Answer from the drawing. Dimensions are ordinates in mm from the lowest x, y and z of the part. A direction names the side the tool comes from. Round coordinates to 2 decimals unless told otherwise and drop trailing zeros. Write each loop counter-clockwise with the first axis right and the second up, starting at its lowest first coordinate (ties: lowest second). Pieces come first, ordered by that corner, then holes. Notation, with made-up numbers: (25, 38) - (84, 38) arc R14 ccw to (84, 46) - close; hole circle Ø5 at (-20.75, 59). An arc over 180 degrees is marked (long way). Answer in a Markdown table with one row per item.
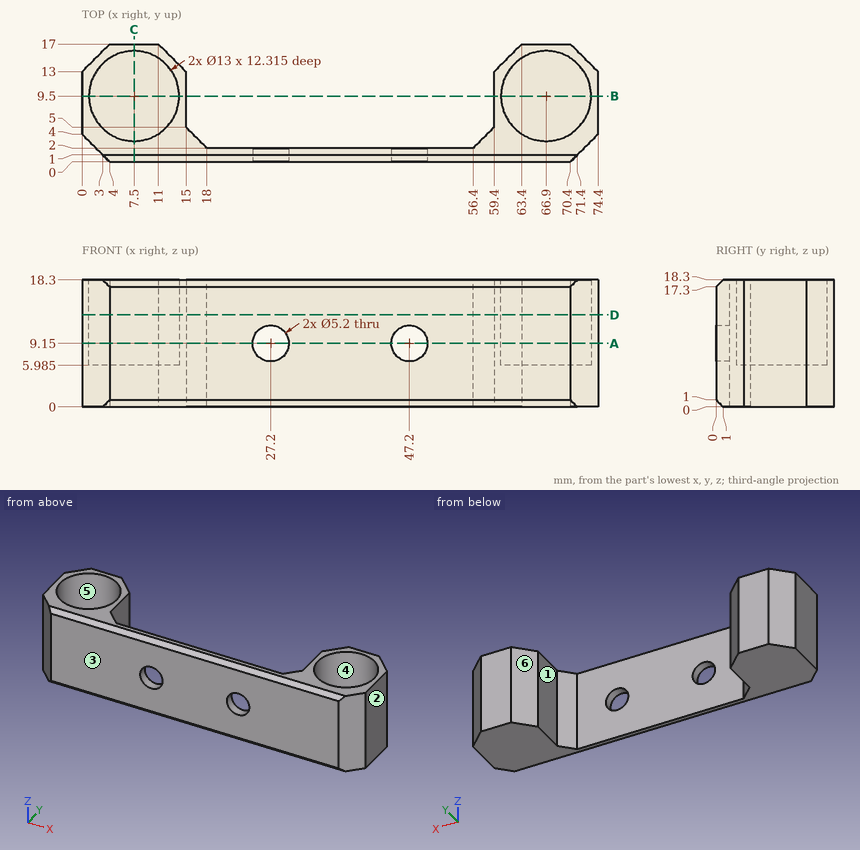
(1) For the marked faces 1 and 2, determine the directions among +Z, -Z, +X, -X, +Y, -Y from which every point of the face is accessible in a straight line to the end or side of a thin tool.
Checked values:
| item | result |
|---|---|
| face 1 | +Z, -Z, +Y |
| face 2 | +Z, -Z, +X, +Y, -Y |
(2) Section D-D (z = 13.25) is taken. Give the vertices of the cut face in (x, y), and give its area (3 significant figures).
Checked values:
| item | result |
|---|---|
| outline | (0, 4) - (4, 0) - (70.4, 0) - (74.4, 4) - (74.4, 13) - (70.4, 17) - (63.4, 17) - (59.4, 13) - (59.4, 5) - (56.4, 2) - (18, 2) - (15, 5) - (15, 13) - (11, 17) - (4, 17) - (0, 13) - close; hole circle Ø13 at (7.5, 9.5); hole circle Ø13 at (66.9, 9.5) |
| area | 294 mm2 |
(3) For a pull along Y with two mould halves and no side action, classify the marked faces 3, 4, 5 and 6 as pulls with the +Y half, pulls with the -Y half, needs draft (parallel to the pull), parting line crosses it, or undercut.
Checked values:
| item | result |
|---|---|
| face 3 | pulls with the -Y half |
| face 4 | undercut |
| face 5 | undercut |
| face 6 | pulls with the +Y half |
(4) Section B-B (y = 9.5) is taken. Give the vertices of the cut face in (x, z) (3 decimals), and give its area (3 significant figures).
Checked values:
| item | result |
|---|---|
| outline | (0, 0) - (15, 0) - (15, 18.3) - (14, 18.3) - (14, 5.985) - (1, 5.985) - (1, 18.3) - (0, 18.3) - close; (59.4, 0) - (74.4, 0) - (74.4, 18.3) - (73.4, 18.3) - (73.4, 5.985) - (60.4, 5.985) - (60.4, 18.3) - (59.4, 18.3) - close |
| area | 229 mm2 |
(5) Section A-A (z = 9.15) is taken. Give the vertices of the cut face in (x, y), and give its area (3 significant figures).
Checked values:
| item | result |
|---|---|
| outline | (0, 4) - (4, 0) - (24.6, 0) - (24.6, 2) - (18, 2) - (15, 5) - (15, 13) - (11, 17) - (4, 17) - (0, 13) - close; (29.8, 0) - (44.6, 0) - (44.6, 2) - (29.8, 2) - close; (49.8, 0) - (70.4, 0) - (74.4, 4) - (74.4, 13) - (70.4, 17) - (63.4, 17) - (59.4, 13) - (59.4, 5) - (56.4, 2) - (49.8, 2) - close; hole circle Ø13 at (7.5, 9.5); hole circle Ø13 at (66.9, 9.5) |
| area | 274 mm2 |
(6) Find the intervals of material crossed by line 1 (X direction, y = 5.5, z = 12); line 2 (X direction, y = 6.25, z = 12.25); line 3 (X direction, y = 0.95, z = 9.15), in increasing order.
Checked values:
| item | result |
|---|---|
| line 1 | x = 0 to 2.38, 12.62 to 15, 59.4 to 61.78, 72.02 to 74.4 |
| line 2 | x = 0 to 1.87, 13.13 to 15, 59.4 to 61.27, 72.53 to 74.4 |
| line 3 | x = 3.05 to 24.6, 29.8 to 44.6, 49.8 to 71.35 |
(7) Section C-C (x = 7.5) is taken. Give the vertices of the cut face in (y, z) (3 decimals), and give its area (3 significant figures).
Checked values:
| item | result |
|---|---|
| outline | (0, 1) - (1, 0) - (17, 0) - (17, 18.3) - (16, 18.3) - (16, 5.985) - (3, 5.985) - (3, 18.3) - (1, 18.3) - (0, 17.3) - close |
| area | 150 mm2 |
(8) Flat-ended cylindrical pins translate along their axes: pin 1 (6.5 mm diameter, centred on x = 69, y = 8, fed in from +Z) (3 decimals); pin 2 (6 mm diameter, centred on x = 57, z = 8.5, fed in from +Y); pin 3 (3 mm diameter, centred on x = 27.2, z = 9.15, fed in from -Y). Find the tip coordinate at first contact, or state that the pin passes through.
Checked values:
| item | result |
|---|---|
| pin 1 | stops at z = 5.985 |
| pin 2 | stops at y = 13.6 |
| pin 3 | passes through |
